from build123d import *

# Parameters (mm, degrees)
SKETCH1_W           = 39.4
SKETCH1_H           = 12
SKETCH1_W_2         = 30.068441065
SKETCH1_H_2         = 1.551330798
BOSS_EXTRUDE2_DEPTH = 1.6
SKETCH2_W           = 5.546376038
SKETCH2_H           = 1.891525972
SKETCH2_W_2         = 8
SKETCH2_H_2         = 1.312065252
BOSS_EXTRUDE4_DEPTH = 1.5
SKETCH5_W           = 5.546376038
SKETCH5_H           = 1.337693851
BOSS_EXTRUDE5_DEPTH = 1.5
SKETCH7_W           = 5.546376038
SKETCH7_H           = 1.5
BOSS_EXTRUDE6_DEPTH = 1.5
SKETCH9_W           = 8
SKETCH9_H           = 1.5
BOSS_EXTRUDE7_DEPTH = 1.5
FILLET3_R           = 1
FILLET4_R           = 1
FILLET5_R           = 1
FILLET6_R           = 1
FILLET7_R           = 0.5


with BuildPart() as part:
    # Sketch1 → Boss-Extrude2 (new body)
    with BuildSketch(Plane(origin=(0, 0, 0), x_dir=(1, 0, 0), z_dir=(0, 1, 0))):
        with Locations((-3.723847257, 0.850254859)):
            Rectangle(SKETCH1_W, SKETCH1_H)
        with Locations((-3.699480126, -2.702390472)):
            Rectangle(SKETCH1_W_2, SKETCH1_H_2, mode=Mode.SUBTRACT)
    extrude(amount=BOSS_EXTRUDE2_DEPTH)

    # Sketch2 → Boss-Extrude4 (add)
    with BuildSketch(Plane(origin=(0, 1.6, 0), x_dir=(1, 0, 0), z_dir=(0, 1, 0))):
        with Locations((-15.450659238, 5.904491873)):
            Rectangle(SKETCH2_W, SKETCH2_H)
        with Locations((8.004202505, 6.017944023)):
            Rectangle(SKETCH2_W, SKETCH2_H)
        with Locations((-4.058606796, -4.493712515)):
            Rectangle(SKETCH2_W_2, SKETCH2_H_2)
    extrude(amount=BOSS_EXTRUDE4_DEPTH)

    # Sketch5 → Boss-Extrude5 (add)
    with BuildSketch(Plane(origin=(0, 0, -6.850254859), x_dir=(-1, 0, 0), z_dir=(0, 0, -1))):
        with Locations((15.450659238, 2.268846926)):
            Rectangle(SKETCH5_W, SKETCH5_H)
    extrude(amount=BOSS_EXTRUDE5_DEPTH)

    # Sketch7 → Boss-Extrude6 (add)
    with BuildSketch(Plane(origin=(0, 0, -6.963707009), x_dir=(-1, 0, 0), z_dir=(0, 0, -1))):
        with Locations((-8.004202505, 2.35)):
            Rectangle(SKETCH7_W, SKETCH7_H)
    extrude(amount=BOSS_EXTRUDE6_DEPTH)

    # Sketch9 → Boss-Extrude7 (add)
    with BuildSketch(Plane.XY.offset(5.149745141)):
        with Locations((-4.058606796, 2.35)):
            Rectangle(SKETCH9_W, SKETCH9_H)
    extrude(amount=BOSS_EXTRUDE7_DEPTH)

    # Fillet3
    fillet3_edges = [part.edges().sort_by_distance(p)[0] for p in [
        (-4.058606796, 3.1, 6.649745141),
    ]]
    fillet(fillet3_edges, radius=FILLET3_R)

    # Fillet4
    fillet4_edges = [part.edges().sort_by_distance(p)[0] for p in [
        (-15.450659238, 2.937693851, -8.350254859),
        (8.004202505, 3.1, -8.463707009),
    ]]
    fillet(fillet4_edges, radius=FILLET4_R)

    # Fillet5
    fillet5_edges = [part.edges().sort_by_distance(p)[0] for p in [
        (8.004202505, 3.1, -5.072181037),
        (-15.450659238, 3.1, -4.958728887),
    ]]
    fillet(fillet5_edges, radius=FILLET5_R)

    # Fillet6
    fillet6_edges = [part.edges().sort_by_distance(p)[0] for p in [
        (-4.058606796, 3.1, 3.837679889),
    ]]
    fillet(fillet6_edges, radius=FILLET6_R)

    # Fillet7
    fillet7_edges = [part.edges().sort_by_distance(p)[0] for p in [
        (-23.423847257, 0.8, -6.850254859),
        (15.976152743, 0.8, -6.850254859),
        (15.976152743, 0.8, 5.149745141),
        (-23.423847257, 0.8, 5.149745141),
    ]]
    fillet(fillet7_edges, radius=FILLET7_R)


solid = part.part
Source: CAD feature listing. Evaluate the final solid. Frame: model axes, mm. A direction names the side the tool comes from. Coordinates: 2 decimals unless noted, no trailing zeros. Loops run counter-clockwise (first coordinate to the right, second up) from the corner with the lowest first, then second, coordinate; pieces in that order, holes last. Notation, with made-up numbers: (46.25, 6.25) - (65.25, 6.25) arc R23 ccw to (65.25, 34.25) - close; hole circle Ø9 at (55, 50). An arc over 180 degrees is marked (long way). Return JSON: item names as keys, results as strings.
Q1. Access query for faces 1 (the cylindrical face through (8.04, 2.8, -5.36)), 2 (the flat face through (-12.677, 2, -7)), 3 (the cylindrical face through (-15.5, 2.6, -8.1)), 4 (the flat face through (11.335, 1, 3)). Directions: +Z, -Z, +X, -X, +Y, -Y. A direction counts if a zero-diameter tool reaches every point of the face in a straight line with its end or side. Return the directions, or none.
Results:
{"face 1": "+Z, +X, +Y", "face 2": "+Z, -Z, +Y", "face 3": "-Z, -X, +Y", "face 4": "+Y, -Y"}
Q2. Section A-A, the plane x = 8.5. Return loops of the section in (y, z), plus the area to 3 significant figures.
Results:
{"outline": "(0, -6.85) - (1.6, -6.85) - (1.6, -8.46) - (2.1, -8.46) arc R1 ccw to (3.1, -7.46) - (3.1, -6.07) arc R1 ccw to (2.1, -5.07) - (1.6, -5.07) - (1.6, 1.93) - (0, 1.93) - close; (0, 3.48) - (1.6, 3.48) - (1.6, 5.15) - (0, 5.15) - close", "area": "21.4 mm2"}
Q3. Contact query for flat-ended pins moving along their axis: P1, Ø5, axis at x = 10, z = -1, coming from the +Y side; P2, Ø0.8, axis at x = 0.5, y = 0.5, coming from the +Z side; P3, Ø0.5, axis at y = 2.5, z = -6.5, coming from the +X side. Output: stop coordinate, or through.
Results:
{"P1": "y = 1.6", "P2": "z = 5.15", "P3": "x = 10.78"}
Q4. Section D-D, the plane x = -17.5. Return loops of the section in (y, z), plus the area to 3 significant figures.
Results:
{"outline": "(0, -6.85) - (1.6, -6.85) - (1.6, -8.35) - (1.94, -8.35) arc R1 ccw to (2.94, -7.35) - (2.94, -6.85) - (3.1, -6.85) - (3.1, -5.96) arc R1 ccw to (2.1, -4.96) - (1.6, -4.96) - (1.6, 1.93) - (0, 1.93) - close; (0, 3.48) - (1.6, 3.48) - (1.6, 5.15) - (0, 5.15) - close", "area": "21.1 mm2"}
Q5. Material intervals for line 1 along Z through (x, y) = (8, 1.1); line 2 along X through (y, z) = (2.7, -6); line 3 along Y through (x, z) = (0, 1.75), sorted ascending.
Results:
{"line 1": "-6.85 to 1.93, 3.48 to 5.15", "line 2": "-18.22 to -12.68, 5.23 to 10.78", "line 3": "0 to 1.6"}
Q6. Section B-B, the plane z = 2.5. Return loops of the section in (x, y), plus the area to 3 significant figures.
Results:
{"outline": "(-23.42, 0) - (-18.73, 0) - (-18.73, 1.6) - (-23.42, 1.6) - close; (11.33, 0) - (15.98, 0) - (15.98, 1.6) - (11.33, 1.6) - close", "area": "14.9 mm2"}
Q7. Section C-C, the plane y = 0.95. Return loops of the section in (x, z).
Results:
{"outline": "(-23.42, -6.35) arc R0.5 ccw to (-22.92, -6.85) - (15.48, -6.85) arc R0.5 ccw to (15.98, -6.35) - (15.98, 4.65) arc R0.5 ccw to (15.48, 5.15) - (-22.92, 5.15) arc R0.5 ccw to (-23.42, 4.65) - close; hole (-18.73, 1.93) - (11.33, 1.93) - (11.33, 3.48) - (-18.73, 3.48) - close"}
Q8. Mould query, pull axis X, two halves, no side actions, for faces 5 (the flat face through (-4, 1, 1.927)), 6 (the flat face through (10.777, 2, -7)), 7 (the flat face through (-4, 1, -6.85)). Classes: released by +X, released by -X, zero draft, split by the parting line, or undercut.
Results:
{"face 5": "undercut", "face 6": "released by +X", "face 7": "zero draft"}
